Could you check a few things on this model? Use its own coordinates, in mm. A direction names the side the tool comes from. Give positions to 0.01 mm unless a question says otherwise; leave off trailing zeros. Loops run counter-clockwise (first coordinate to the right, second up) from the corner with the lowest first, then second, coordinate; pieces in that order, holes last. Notation, with made-up numbers: (-16.75, 63) - (11.25, 63) arc R32 cw to (11.25, 89) - close; hole circle Ø3 at (-21, 65.25). An arc over 180 degrees is marked (long way). Use CSV: the item, a comma, the result in double quotes.
from build123d import *

# Parameters (mm, degrees)
SKETCH1_W           = 7.4
SKETCH1_H           = 11.5
BOSS_EXTRUDE1_DEPTH = 5.7
SKETCH2_R           = 2.5
CUT_EXTRUDE1_DEPTH  = 5.5
SKETCH3_R           = 1
BOSS_EXTRUDE2_DEPTH = 5.5
SKETCH4_R           = 0.25
CUT_EXTRUDE2_DEPTH  = 5.5
SKETCH5_W           = 4.2
SKETCH5_H           = 1
BOSS_EXTRUDE3_DEPTH = 4.5
FILLET1_R           = 1
CUT_EXTRUDE3_REACH  = 5.5
SKETCH6_R           = 1


with BuildPart() as part:
    # Sketch1 → Boss-Extrude1 (new body)
    with BuildSketch(Plane(origin=(0, 0, 0), x_dir=(1, 0, 0), z_dir=(0, 1, 0))):
        with Locations((3.7, 5.75)):
            Rectangle(SKETCH1_W, SKETCH1_H)
    extrude(amount=BOSS_EXTRUDE1_DEPTH)

    # Sketch2 → Cut-Extrude1 (cut)
    with BuildSketch(Plane.XY):
        with Locations((3.7, 2.85)):
            Circle(SKETCH2_R)
    extrude(amount=-CUT_EXTRUDE1_DEPTH, mode=Mode.SUBTRACT)

    # Sketch3 → Boss-Extrude2 (add)
    with BuildSketch(Plane.XY):
        with Locations((3.7, 2.85)):
            Circle(SKETCH3_R)
    extrude(amount=-BOSS_EXTRUDE2_DEPTH)

    # Sketch4 → Cut-Extrude2 (cut)
    with BuildSketch(Plane.XY):
        with Locations((3.7, 2.85)):
            Circle(SKETCH4_R)
    extrude(amount=-CUT_EXTRUDE2_DEPTH, mode=Mode.SUBTRACT)

    # Sketch5 → Boss-Extrude3 (add)
    with BuildSketch(Plane(origin=(7.4, 0, 0), x_dir=(0, 0, -1), z_dir=(1, 0, 0))):
        with Locations((5.6, 3)):
            Rectangle(SKETCH5_W, SKETCH5_H)
    extrude(amount=BOSS_EXTRUDE3_DEPTH)

    # Fillet1
    fillet1_edges = [part.edges().sort_by_distance(p)[0] for p in [
        (11.9, 3, -3.5),
        (11.9, 3, -7.7),
    ]]
    fillet(fillet1_edges, radius=FILLET1_R)

    # Sketch6 → Cut-Extrude3 (cut, up to next)
    with BuildSketch(Plane(origin=(0, 3.5, 0), x_dir=(1, 0, 0), z_dir=(0, 1, 0)), mode=Mode.PRIVATE) as cut_extrude3_sk1:
        with Locations((9.9, 5.5)):
            Circle(SKETCH6_R)
    cut_extrude3_tool1 = extrude(cut_extrude3_sk1.sketch, amount=-CUT_EXTRUDE3_REACH, mode=Mode.PRIVATE) & part.part
    add(cut_extrude3_tool1.solids().sort_by_distance((9.9, 3.5, -5.5))[0], mode=Mode.SUBTRACT)


solid = part.part
1) I need wall thicknesses on line 1 along Y through (x, z) = (3.7, -3.1); line 2 along Z through (x, y) = (9.9, 3); line 3 along X through (y, z) = (1.45, -1.25). Which ranges of each line are inside material? Lowest first, please.
Answer below:
line 1,"y = 0 to 0.35, 1.85 to 2.6, 3.1 to 3.85, 5.35 to 5.7"
line 2,"z = -7.7 to -6.5, -4.5 to -3.5"
line 3,"x = 0 to 1.63, 5.77 to 7.4"
2) Suppose I cut it at D-D (y = 1.2). Please give me the cut outline in (x, z).
Answer below:
outline,"(0, -11.5) - (7.4, -11.5) - (7.4, 0) - (5.58, 0) - (5.58, -5.5) - (1.82, -5.5) - (1.82, 0) - (0, 0) - close"
3) Suppose I cut it at B-B (x = 3.7). Please give me the cut outline in (y, z).
Answer below:
outline,"(0, -11.5) - (5.7, -11.5) - (5.7, 0) - (5.35, 0) - (5.35, -5.5) - (3.85, -5.5) - (3.85, 0) - (3.1, 0) - (3.1, -5.5) - (2.6, -5.5) - (2.6, 0) - (1.85, 0) - (1.85, -5.5) - (0.35, -5.5) - (0.35, 0) - (0, 0) - close"
4) Suppose I cut it at C-C (y = 2.85). Please give me the cut outline in (x, z).
Answer below:
outline,"(0, -11.5) - (7.4, -11.5) - (7.4, -7.7) - (10.9, -7.7) arc R1 ccw to (11.9, -6.7) - (11.9, -4.5) arc R1 ccw to (10.9, -3.5) - (7.4, -3.5) - (7.4, 0) - (6.2, 0) - (6.2, -5.5) - (4.7, -5.5) - (4.7, 0) - (3.95, 0) - (3.95, -5.5) - (3.45, -5.5) - (3.45, 0) - (2.7, 0) - (2.7, -5.5) - (1.2, -5.5) - (1.2, 0) - (0, 0) - close; hole circle Ø2 at (9.9, -5.5)"
5) Which directions (+Z, -Z, +X, -X, +Y, -Y) give clear straight access to the entire face, cutting with the end or side of a thin tool? Please do faces 4 (the flat face through (8.6, 3.5, -5.6)), 5 (the flat face through (9, 3, -7.7)), 6 (the flat face through (9, 3, -3.5)).
Answer below:
face 4,"+Z, -Z, +X, +Y"
face 5,"-Z, +X, +Y, -Y"
face 6,"+Z, +X, +Y, -Y"
6) We'd pull the mould along Y, two halves only. Please class faces 1 (the cylindrical face through (5.04, 4.96, -2.71)), 2 (the flat face through (4, 5.7, -6)), 3 (the flat face through (0, 3, -6)): +Y half, -Y half, draft (parallel to the pull), parting line (faces both ways), or undercut.
Answer below:
face 1,"undercut"
face 2,"+Y half"
face 3,"draft"
7) I'm going to push flat-ended pins straight in: P1, Ø0.5, axis at x = 9, y = 3, coming from the -Z side; P2, Ø3.5, axis at x = 9.5, z = -5, coming from the +Y side. Where does each tip first touch, or does it pass through?
Answer below:
P1,"stops at z = -7.7"
P2,"stops at y = 3.5"
8) Suppose I cut it at A-A (x = 9.9). Please give me the cut outline in (y, z).
Answer below:
outline,"(2.5, -7.7) - (3.5, -7.7) - (3.5, -6.5) - (2.5, -6.5) - close; (2.5, -4.5) - (3.5, -4.5) - (3.5, -3.5) - (2.5, -3.5) - close"
